from build123d import *

# Parameters (mm, degrees)
SKETCH1_R           = 6.35
BOSS_EXTRUDE1_DEPTH = 50.8
CIRPATTERN1_COUNT   = 2
CIRPATTERN1_ANGLE   = 90


with BuildPart() as part:
    # Sketch1 → Boss-Extrude1 (new body)
    with BuildSketch(Plane.XY):
        Circle(SKETCH1_R)
    boss_extrude1 = extrude(amount=BOSS_EXTRUDE1_DEPTH)

    # CirPattern1: Boss-Extrude1 ×2 about axis
    cirpattern1_axis = Axis((0, 6.35, 25.4), (0, -1, 0))
    for i in range(1, CIRPATTERN1_COUNT):
        add(boss_extrude1.rotate(cirpattern1_axis, i * CIRPATTERN1_ANGLE / (CIRPATTERN1_COUNT - 1)))


solid = part.part
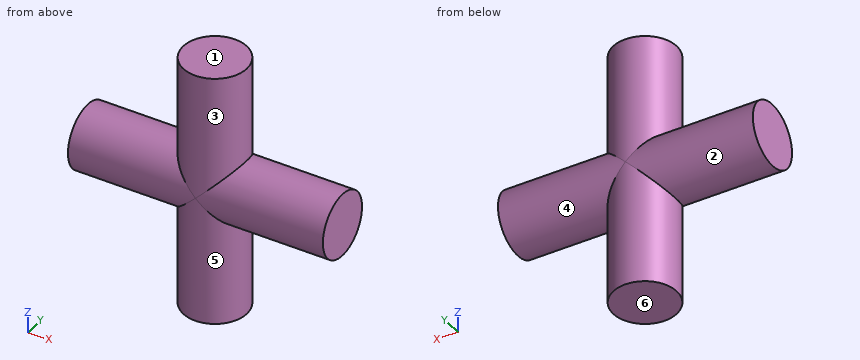
Geometry check sheet. Reference: the model listing, model coordinates, mm. Face numbers are marked on the shaded views. A direction names the side the tool comes from. Round coordinates to 2 decimals unless told otherwise and drop trailing zeros. Order: outer loops, then holes, each group sorted by start corner. A loop starts at its lowest first (then second) coordinate and runs counter-clockwise, first axis right, second up. Notation, with made-up numbers: (51, 60) - (102, 60) arc R28 cw to (102, 84) - close; hole circle Ø3 at (-34, 57). An arc over 180 degrees is marked (long way). One line per question, with ' | ' between items. Start each with the question number.
(1) Release check for a two-part mould opening along Z. For the marked faces 1, 2 and 3 record: released by +Z, released by -Z, zero draft, split by the parting line, or undercut.
(2) Sectioned sample at A-A on y = 4.25. Record the cut outline in (x, z), and give its area (3 significant figures).
(3) Thickness scan on L1, parallel to Z at x = 9, y = 3; L2, parallel to X at y = -3.25, z = 34; L3, parallel to Y at x = -18.5, z = 25.5. Record the ranges inside material, lowest first. Write a range as [from, to].
(4) Sectioned sample at D-D on y = 0. Record the cut outline in (x, z), and give its area (3 significant figures).
(5) Depth check by flat-ended pin: pin 1 Ø3 at (y, z) = (2.5, 43) entering from -X; pin 2 Ø4 at (x, y) = (9.5, 3.5) entering from -Z; pin 3 Ø6 at (y, z) = (5, 6.5) entering from +X; pin 4 Ø5 at (x, z) = (9, 43.5) entering from -Y. Enter the tip coordinate at first touch or a pass-through.
(6) Sectioned sample at B-B on z = 22. Record the cut outline in (x, y), and give its area (3 significant figures).
(7) Sectioned sample at C-C on x = -20. Record the cut outline in (y, z).
(8) Access from +Z, -Z, +X, -X, +Y, -Y to the whole of each face (thin tool, end or side, straight path). Record for the marked faces 4, 5 and 6.
Conclusion:
1) face 1: released by +Z | face 2: split by the parting line | face 3: zero draft
2) outline: (-25.4, 20.68) - (-4.72, 20.68) - (-4.72, 0) - (4.72, 0) - (4.72, 20.68) - (25.4, 20.68) - (25.4, 30.12) - (4.72, 30.12) - (4.72, 50.8) - (-4.72, 50.8) - (-4.72, 30.12) - (-25.4, 30.12) - close | area: 870 mm2
3) L1: z = [19.8, 31] | L2: x = [-5.46, 5.46] | L3: y = [-6.35, 6.35]
4) outline: (-25.4, 19.05) - (-6.35, 19.05) - (-6.35, 0) - (6.35, 0) - (6.35, 19.05) - (25.4, 19.05) - (25.4, 31.75) - (6.35, 31.75) - (6.35, 50.8) - (-6.35, 50.8) - (-6.35, 31.75) - (-25.4, 31.75) - close | area: 1,130 mm2
5) pin 1: stops at x = -6.27 | pin 2: stops at z = 19.23 | pin 3: stops at x = 6.03 | pin 4: passes through
6) outline: (-25.4, -5.36) - (-3.4, -5.36) arc R6.35 ccw to (3.4, -5.36) - (25.4, -5.36) - (25.4, 5.36) - (3.4, 5.36) arc R6.35 ccw to (-3.4, 5.36) - (-25.4, 5.36) - close | area: 554 mm2
7) outline: circle Ø12.7 at (0, 25.4)
8) face 4: +X | face 5: -Z | face 6: -Z, +X, -X, +Y, -Y
